Read the model definition and answer for the solid it produces. Units are mm, in the model's axes. Face numbers are marked on the shaded views. A direction names the side the tool comes from. Give positions to 0.01 mm unless a question says otherwise; leave off trailing zeros. Loops run counter-clockwise (first coordinate to the right, second up) from the corner with the lowest first, then second, coordinate; pieces in that order, holes last. Notation, with made-up numbers: (11, 0.5) - (48, 0.5) arc R35 ccw to (48, 37.5) - close; hole circle Ø5 at (-25.5, 83). An arc over 180 degrees is marked (long way). Write item = value, one per line. Start each with the question number.
Autodesk Inventor part; units mm, degrees
ref_plane "bracket_to_dummy_XY" through (0, 0, 0) normal (0, 1, 0) x (1, 0, 0)
ref_plane "bracket_to_dummy_YZ" through (0, 0, 0) normal (1, 0, 0) x (0, 0, -1)
ref_plane "bracket_to_dummy_ZX" through (0, 0, 0) normal (0, 0, -1) x (0, 1, 0)
sketch "Sketch_1" plane through (0, 0, 0) normal (1, 0, 0) x (0, 1, 0)
  line L0 (0, 80) -> (0, 0)
  line L1 (0, 0) -> (56.5685, 56.5685)
  line L2 (56.5685, 56.5685) -> (50.2046, 62.9325)
  line L3 (50.2046, 62.9325) -> (36.0624, 48.7904)
  line L4 (36.0624, 48.7904) -> (9, 60)
  line L5 (9, 60) -> (9, 80)
  line L6 (9, 80) -> (0, 80)
  arc A0 (6.8931, 25.3806) -> (5, 23.933) centre (6.5, 23.933) ccw
  line L7 (5, 23.933) -> (5, 15.6924)
  arc A1 (5, 15.6924) -> (7.5607, 14.6317) centre (6.5, 15.6924) ccw
  line L8 (7.5607, 14.6317) -> (13.3877, 20.4587)
  arc A2 (13.3877, 20.4587) -> (13.0726, 22.821) centre (12.327, 21.5194) ccw
  arc A3 (13.0726, 22.821) -> (6.8931, 25.3806) centre (0, 0) ccw
  circle A4 centre (12, 28.9706) radius 2.1
  arc A5 (7.074, 56.4682) -> (5, 55.0824) centre (6.5, 55.0824) ccw
  line L9 (5, 55.0824) -> (5, 32.7559)
  arc A6 (5, 32.7559) -> (7.5929, 31.7285) centre (6.5, 32.7559) ccw
  line L10 (7.5929, 31.7285) -> (8.2843, 32.4639)
  arc A7 (17.0976, 28.8133) -> (8.2843, 32.4639) centre (12, 28.9706) ccw
  line L11 (17.0976, 28.8133) -> (17.0665, 27.8044)
  arc A8 (17.0665, 27.8044) -> (19.6264, 26.6975) centre (18.5657, 27.7581) ccw
  line L12 (19.6264, 26.6975) -> (35.4136, 42.4847)
  arc A9 (35.4136, 42.4847) -> (34.927, 44.9311) centre (34.3529, 43.5453) ccw
  line L13 (34.927, 44.9311) -> (7.074, 56.4682)
extrude "Extrusion1" add sketch "Sketch_1" along normal mid plane 14
sketch "Sketch2" plane through (-7, 50.2046, 62.9325) normal (0, -0.7071068, 0.7071068) x (1, 0, 0)
  point P0 (7, -10)
hole "Hole1" at (0, 43.1335, 55.8614) direction (0, 0.7071068, -0.7071068) diameter 5.5 depth 9
sketch "Sketch3" plane through (-7, 0, 80) normal (0, -1, 0) x (1, 0, 0)
  point P0 (7, -10)
hole "Hole2" at (0, 0, 70) direction (0, 1, 0) diameter 5.5 depth 9
ref_plane "bracket_to_dummy_XY" through (0, 0, 0) normal (0, 1, 0) x (1, 0, 0)
ref_plane "bracket_to_dummy_YZ" through (0, 0, 0) normal (1, 0, 0) x (0, 0, -1)
ref_plane "bracket_to_dummy_ZX" through (0, 0, 0) normal (0, 0, -1) x (0, 1, 0)
ref_plane "to_bolts_b_1_XY" through (0, 43.1335, 55.8614) normal (0, -0.7071068, 0.7071068) x (1, 0, 0)
ref_plane "to_bolts_b_1_YZ" through (0, 43.1335, 55.8614) normal (1, 0, 0) x (0, 0.7071068, 0.7071068)
ref_plane "to_bolts_b_1_ZX" through (0, 43.1335, 55.8614) normal (0, 0.7071068, 0.7071068) x (0, -0.7071068, 0.7071068)
ref_plane "to_bolts_base_b_1_XY" through (0, 9, 70) normal (0, 1, 0) x (1, 0, 0)
ref_plane "to_bolts_base_b_1_YZ" through (0, 9, 70) normal (1, 0, 0) x (0, 0, -1)
ref_plane "to_bolts_base_b_1_ZX" through (0, 9, 70) normal (0, 0, -1) x (0, 1, 0)
ref_plane "to_nuts_b_1_XY" through (0, 50.9117, 48.0833) normal (0, -0.7071068, 0.7071068) x (1, 0, 0)
ref_plane "to_nuts_b_1_YZ" through (0, 50.9117, 48.0833) normal (1, 0, 0) x (0, 0.7071068, 0.7071068)
ref_plane "to_nuts_b_1_ZX" through (0, 50.9117, 48.0833) normal (0, 0.7071068, 0.7071068) x (0, -0.7071068, 0.7071068)
ref_plane "to_nuts_base_b_1_XY" through (0, -2, 70) normal (0, 1, 0) x (1, 0, 0)
ref_plane "to_nuts_base_b_1_YZ" through (0, -2, 70) normal (1, 0, 0) x (0, 0, -1)
ref_plane "to_nuts_base_b_1_ZX" through (0, -2, 70) normal (0, 0, -1) x (0, 1, 0)
properties part number "HBL45TS5hbl45ts5" material "Stainless Steel"
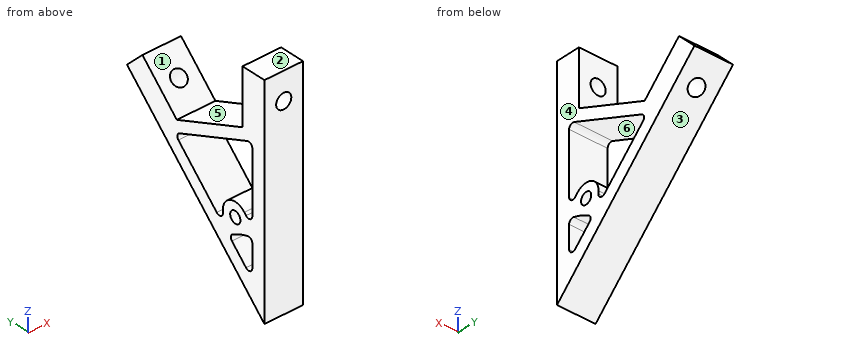
1. A tool of negligible diameter and unlimited length cuts with its end or side. For the marked faces 4, 5 and 6, from which of +Z, -Z, +X, -X, +Y, -Y can it reach the whole face along a straight path? Write none if from no direction.
2. A cutting plane is placed at D-D on y = 12. Give the vertices of the cut face in (x, z), and give its area (3 significant figures).
3. A cutting plane is placed at C-C on y = 29. Give the vertices of the cut face in (x, z).
4. Consider line 1 along Y through (x, z) = (-6.5, 55); line 2 along X through (y, z) = (5, 70); line 3 along Z through (x, y) = (3.5, 12). Determine where each line is inside the solid, lowest interval first. Write a range as [from, to].
5. Given P1, Ø4, axis at x = -2.5, z = 18.5, coming from the +Y side; P2, Ø6, axis at x = -4.5, z = 12.5, coming from the +Y side; P3, Ø6, axis at x = -5.5, y = 11, coming from the +Z side; P4, Ø7, axis at x = 0.5, z = 74.5, coming from the +Y side, each flat-ended and moving along its own axis, determine where each tip first touches the part or whether it passes through.
6. A cutting plane is placed at A-A on z = 70. Give the vertices of the cut face in (x, y).
7. For a pull along Y with two mould halves and no side action, classify the marked faces 1, 2 and 3 as released by +Y, released by -Y, zero draft, split by the parting line, or undercut.
8. A cutting plane is placed at B-B on x = 0. Give the number of separate pieces and of enclosed holes in the cut face, and give its area (3 significant figures).
Reply:
q1.face_4 = +Z, -Z, +X, +Y, -Y
q1.face_5 = +Z, +X, -X
q1.face_6 = +X, -X
q2.outline = (-7, 12) - (7, 12) - (7, 19.07) - (-7, 19.07) - close; (-7, 23.4) - (7, 23.4) - (7, 26.87) - (-7, 26.87) - close; (-7, 31.07) - (7, 31.07) - (7, 34.07) - (-7, 34.07) - close; (-7, 54.43) - (7, 54.43) - (7, 58.76) - (-7, 58.76) - close
q2.area = 250 mm^2
q3.outline = (-7, 29) - (7, 29) - (7, 36.07) - (-7, 36.07) - close; (-7, 47.39) - (7, 47.39) - (7, 51.72) - (-7, 51.72) - close
q4.line_1 = [0, 5], [10.62, 21.07], [42.27, 55]
q4.line_2 = [-7, -2.75], [2.75, 7]
q4.line_3 = [12, 19.07], [23.4, 26.87], [31.07, 34.07], [54.43, 58.76]
q5.P1 = 20.5
q5.P2 = 15.5
q5.P3 = 80
q5.P4 = 9
q6.outline = (-7, 0) - (-2.75, 0) - (-2.75, 9) - (-7, 9) - close; (2.75, 0) - (7, 0) - (7, 9) - (2.75, 9) - close
q7.face_1 = undercut
q7.face_2 = zero draft
q7.face_3 = released by +Y
q8.separate_pieces = 3
q8.enclosed_holes = 3
q8.area = 1,040 mm^2
